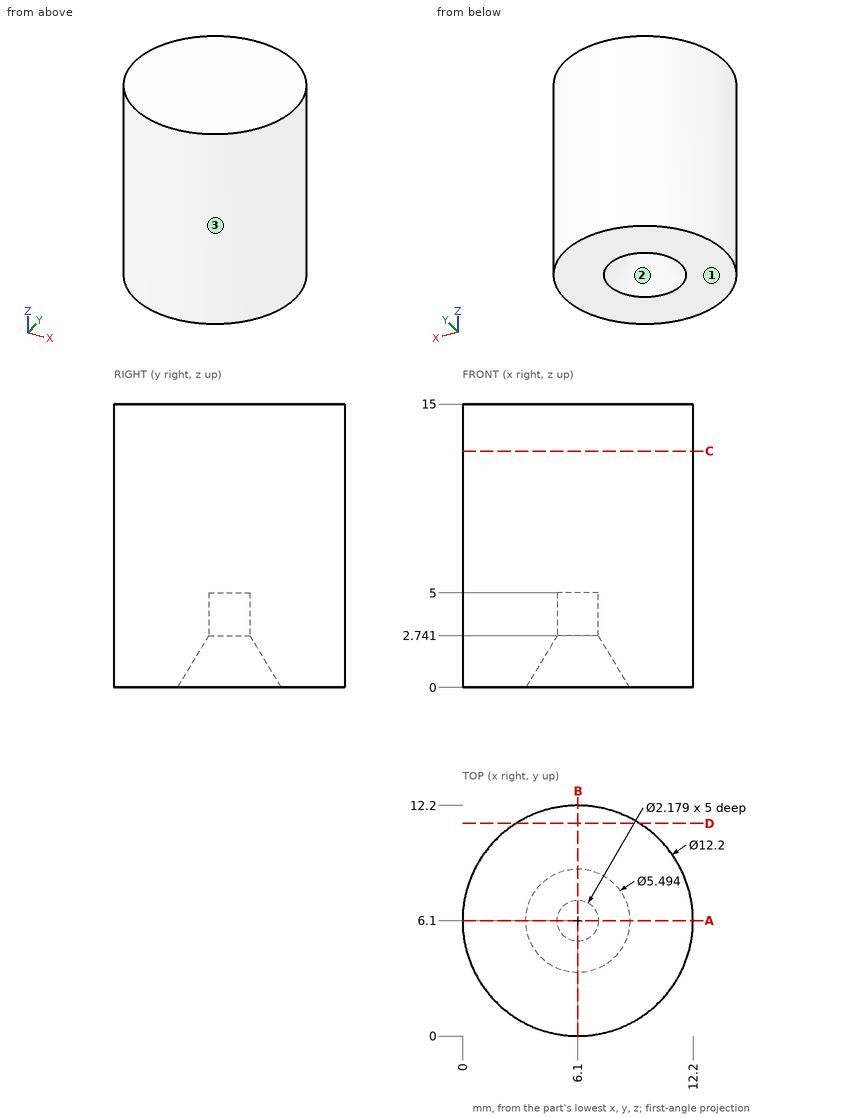
Check sheet for the drawn part. Datum: minimum x, y, z corner. Units: mm. Round coordinates to 2 decimals unless told otherwise and drop trailing zeros. Order: outer loops, then holes, each group sorted by start corner. A loop starts at its lowest first (then second) coordinate and runs counter-clockwise, first axis right, second up. Notation, with made-up numbers: M -9,41.25 L 31,41.25 A18 ccw 31,46.25 Z; hole C 9,48 d8. An arc over 180 degrees is marked long. Answer in a Markdown table with one row per item.
(1) Section check C-C on z = 12.5. Record the boundary of the cut face in (x, y), plus the area to 3 significant figures.
Findings:
| item | result |
|---|---|
| outline | C 6.1,6.1 d12.2 |
| area | 117 mm^2 |
(2) Gauge pin test, flat ends, axial feed: pin 1 (1.5 mm diameter, centred on x = 3, z = 1.5, fed in from +Y); pin 2 (1 mm diameter, centred on y = 3.5, z = 13, fed in from +X); pin 3 (2 mm diameter, centred on x = 8.5, y = 9.5, fed in from -Z); pin 4 (2 mm diameter, centred on x = 10.5, z = 8, fed in from -Y) (1 decimal). Record the tip position at first contact, or that the pin passes through.
Findings:
| item | result |
|---|---|
| pin 1 | stops at y = 11.73 |
| pin 2 | stops at x = 11.83 |
| pin 3 | stops at z = 0 |
| pin 4 | stops at y = 1 |
(3) Material ranges on line 1 along Y through (x, z) = (6.1, 3.95); line 2 along X through (y, z) = (5.25, 2.25) (1 decimal); line 3 along X through (y, z) = (1.25, 4.75), recorded low to high. Write a range as from..to.
Findings:
| item | result |
|---|---|
| line 1 | y = 0..5.01, 7.19..12.2 |
| line 2 | x = 0.1..5, 7.2..12.1 |
| line 3 | x = 2.4..9.8 |
(4) Draft check along Y on the marked faces 1, 2 and 3. Enter one of: +Y half, -Y half, draft (parallel to the pull), parting line (faces both ways), or undercut.
Findings:
| item | result |
|---|---|
| face 1 | draft |
| face 2 | undercut |
| face 3 | parting line |
(5) Section check D-D on y = 11.25. Record the boundary of the cut face in (x, z).
Findings:
| item | result |
|---|---|
| outline | M 2.83,0 L 9.37,0 L 9.37,15 L 2.83,15 Z |
(6) Section check A-A on y = 6.1. Record the boundary of the cut face in (x, z).
Findings:
| item | result |
|---|---|
| outline | M 0,0 L 3.35,0 L 5.01,2.74 L 5.01,5 L 7.19,5 L 7.19,2.74 L 8.85,0 L 12.2,0 L 12.2,15 L 0,15 Z |
